CAD build for the part. Positions are in the model's coordinates, mm. Face numbers are marked on the shaded views. A direction names the side the tool comes from. Give positions to 0.01 mm unless a question says otherwise; leave off trailing zeros. Loops run counter-clockwise (first coordinate to the right, second up) from the corner with the lowest first, then second, coordinate; pieces in that order, holes last.
Item 1: Which spindle directions (+Z, -Z, +X, -X, +Y, -Y) get a long thin tool onto all of the face, cutting with end or side? Do the marked faces 1 and 2. Say none if no direction does.
Item 2: Saw through at B-B on x = -9.75. Give the cut face in (y, z).
Item 3: Saw through at A-A on z = 4. Give the cut face in (x, y), plus the area to 3 significant figures.
Item 4: Drop flat-ended pins along their axis: P1, Ø7.5, axis at x = -2.5, z = 4.5, coming from the -Y side; P2, Ø1.9, axis at x = -1, y = 7.5, coming from the +Z side; P3, Ø0.5, axis at y = 7, z = -0.5, coming from the -X side; P4, Ø3.5, axis at x = -6.5, y = 4, coming from the +Z side. Give the stop position or say it passes through.
Item 5: Probe probe 1 along Y at (x, z) = (-4.25, 4); probe 2 along Z at (x, y) = (7.25, 1); probe 3 along Y at (x, z) = (10.5, 7.75). List the from-to ranges inside material, lowest first.
Item 6: Saw through at D-D on y = 2. Give the cut face in (x, z), plus the area to 3 significant figures.
Item 7: Mould opens along Y. For the marked faces 3, 4 and 5 say: released by +Y, released by -Y, zero draft, split by the parting line, or undercut.
Item 8: Saw through at C-C on z = -1.75. Give the cut face in (x, y), plus the area to 3 significant figures.
from build123d import *

# Parameters (mm, degrees)
SKETCH1_W           = 29.3624
SKETCH1_H           = 12.6
BOSS_EXTRUDE1_DEPTH = 8.21
SKETCH4_W           = 29.3624
SKETCH4_H           = 6.51
CUT_EXTRUDE2_DEPTH  = 6.6
BOSS_EXTRUDE2_START = -12.6
SKETCH2_W           = 25.4
SKETCH2_H           = 0.2
BOSS_EXTRUDE2_DEPTH = 14.6
SKETCH3_W           = 1.9812
SKETCH3_H           = 12.6
CUT_EXTRUDE1_DEPTH  = 1.7


with BuildPart() as part:
    # Sketch1 → Boss-Extrude1 (new body)
    with BuildSketch(Plane(origin=(0, 0, 0), x_dir=(1, 0, 0), z_dir=(0, 1, 0))):
        Rectangle(SKETCH1_W, SKETCH1_H)
    extrude(amount=BOSS_EXTRUDE1_DEPTH)

    # Sketch4 → Cut-Extrude2 (cut)
    with BuildSketch(Plane.XY.offset(6.3)):
        with Locations((0, 3.255)):
            Rectangle(SKETCH4_W, SKETCH4_H)
    extrude(amount=-CUT_EXTRUDE2_DEPTH, mode=Mode.SUBTRACT)

    # Sketch2 → Boss-Extrude2 (add)
    with BuildSketch(Plane.XY.offset(6.3).offset(BOSS_EXTRUDE2_START)):
        with Locations((0, 4.51)):
            Rectangle(SKETCH2_W, SKETCH2_H)
    extrude(amount=BOSS_EXTRUDE2_DEPTH)

    # Sketch3 → Cut-Extrude1 (cut)
    with BuildSketch(Plane(origin=(0, 8.21, 0), x_dir=(1, 0, 0), z_dir=(0, 1, 0))):
        with Locations((-13.6906, 0)):
            Rectangle(SKETCH3_W, SKETCH3_H)
        with Locations((13.6906, 0)):
            Rectangle(SKETCH3_W, SKETCH3_H)
    extrude(amount=-CUT_EXTRUDE1_DEPTH, mode=Mode.SUBTRACT)


solid = part.part
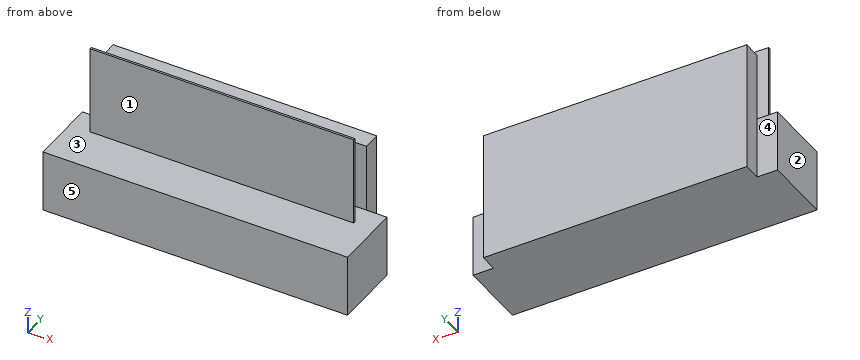
Results below:
1. face 1: +Z, +X, -X, -Y
1. face 2: +Z, -Z, -X, +Y, -Y
2. outline: (0, -6.3) - (8.21, -6.3) - (8.21, 6.3) - (6.51, 6.3) - (6.51, -0.3) - (4.61, -0.3) - (4.61, 8.3) - (4.41, 8.3) - (4.41, -0.3) - (0, -0.3) - close
3. outline: (-12.7, 4.41) - (12.7, 4.41) - (12.7, 4.61) - (-12.7, 4.61) - close; (-12.7, 6.51) - (12.7, 6.51) - (12.7, 8.21) - (-12.7, 8.21) - close
3. area: 48.3 mm2
4. P1: stops at y = 4.41
4. P2: stops at z = 6.3
4. P3: stops at x = -12.7
4. P4: stops at z = 8.3
5. probe 1: y = 4.41 to 4.61, 6.51 to 8.21
5. probe 2: z = -6.3 to -0.3
5. probe 3: y = 4.41 to 4.61
6. outline: (-14.68, -6.3) - (14.68, -6.3) - (14.68, -0.3) - (-14.68, -0.3) - close
6. area: 176 mm2
7. face 3: undercut
7. face 4: released by +Y
7. face 5: released by -Y
8. outline: (-14.68, 0) - (14.68, 0) - (14.68, 6.51) - (12.7, 6.51) - (12.7, 8.21) - (-12.7, 8.21) - (-12.7, 6.51) - (-14.68, 6.51) - close
8. area: 234 mm2
